Source: three-view drawing plus pictorial views. Frame: mm from the lowest corner of the part. A direction names the side the tool comes from. Coordinates: 2 decimals unless noted, no trailing zeros. Order: outer loops, then holes, each group sorted by start corner. A loop starts at its lowest first (then second) coordinate and runs counter-clockwise, first axis right, second up. Notation, with made-up numbers: (36.5, 64) - (51.5, 64) arc R10 ccw to (51.5, 81) - close; hole circle Ø11 at (72.25, -18.75). An arc over 180 degrees is marked (long way). Use a Markdown table: item, result. Add a question column.
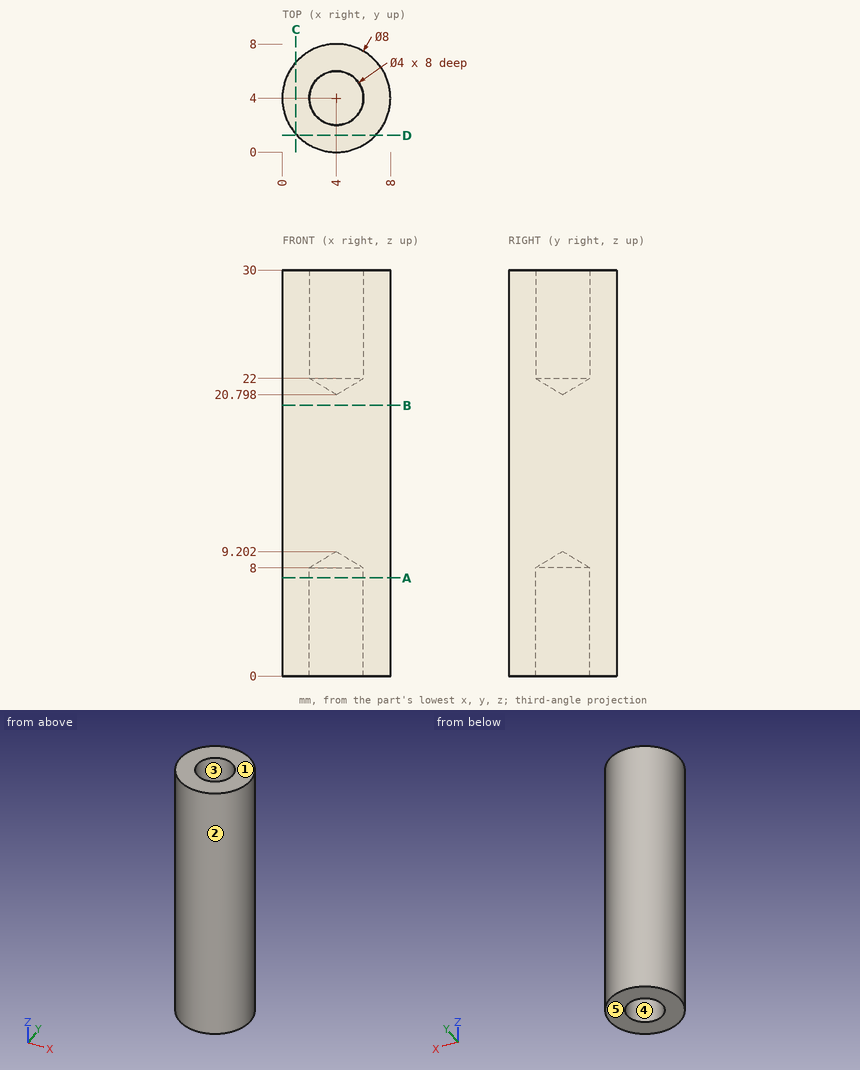
1) Section B-B (z = 20). Return loops of the section in (x, y), then the cut area to 3 significant figures.
2) Draft query along Y for the marked faces 1, 2 and 3. Return one class per face: pulls with the +Y half, pulls with the -Y half, needs draft (parallel to the pull), parting line crosses it, or undercut.
3) Set-up query: the marked faces 4 and 5. Return all of +Z, -Z, +X, -X, +Y, -Y with unobstructed straight access to the full face (end or side cutting, diameter ignored); none if empty.
4) Section C-C (x = 1). Return loops of the section in (y, z), then the cut area to 3 significant figures.
5) Section D-D (y = 1.25). Return loops of the section in (x, z) (1 decimal), then the cut area to 3 significant figures.
6) Section A-A (z = 7.25). Return loops of the section in (x, y), then the cut area to 3 significant figures.
7) Ray query, line 1 along Y through (x, z) = (4, 2.25); line 2 along Y through (x, z) = (5.75, 22.25) (1 decimal). Return the intervals inside material, ascending.
8) Pin query (flat end, axial travel): pin 1 (2.5 mm diameter, centred on x = 4, y = 4, fed in from -Z). Return the tip coordinate at first contact, or that it passes through.
Values follow:
| question | item | result |
|---|---|---|
| 1 | outline | circle Ø8 at (4, 4) |
| 1 | area | 50.3 mm² |
| 2 | face 1 | needs draft |
| 2 | face 2 | parting line crosses it |
| 2 | face 3 | undercut |
| 3 | face 4 | -Z |
| 3 | face 5 | -Z, +X, -X, +Y, -Y |
| 4 | outline | (1.35, 0) - (6.65, 0) - (6.65, 30) - (1.35, 30) - close |
| 4 | area | 159 mm² |
| 5 | outline | (1.1, 0) - (6.9, 0) - (6.9, 30) - (1.1, 30) - close |
| 5 | area | 174 mm² |
| 6 | outline | circle Ø8 at (4, 4); hole circle Ø4 at (4, 4) |
| 6 | area | 37.7 mm² |
| 7 | line 1 | y = 0 to 2, 6 to 8 |
| 7 | line 2 | y = 0.4 to 3, 5 to 7.6 |
| 8 | pin 1 | stops at z = 8.45 |
